Verification items for the finished model (mm, model axes). Face numbers are marked on the shaded views. A direction names the side the tool comes from. Round coordinates to 2 decimals unless told otherwise and drop trailing zeros. Order: outer loops, then holes, each group sorted by start corner. A loop starts at its lowest first (then second) coordinate and runs counter-clockwise, first axis right, second up. Notation, with made-up numbers: M 64,51.25 L 115,51.25 A17 cw 115,60.25 Z; hole C -3.5,80.25 d9. An arc over 180 degrees is marked long. One line per item, written item: value. Start each with the question number.
from build123d import *

# Parameters (mm, degrees)
SKETCH1_W           = 203.2
SKETCH1_H           = 114.3
BOSS_EXTRUDE1_DEPTH = 119.38
SHELL1_T            = -2.54
SKETCH2_R           = 18.5
SKETCH2_R_2         = 2.032
SKETCH2_R_3         = 11.176
CUT_EXTRUDE1_DEPTH  = 2.54
SKETCH3_W           = 114.3
SKETCH3_H           = 119.38
SKETCH3_R           = 18.5
SKETCH3_R_2         = 2.032
SKETCH3_R_3         = 11.176
BOSS_EXTRUDE3_DEPTH = 7.62
SKETCH4_R           = 15.875
CUT_EXTRUDE2_DEPTH  = 2.54
SKETCH5_W           = 50.7
SKETCH5_H           = 7.62
BOSS_EXTRUDE4_DEPTH = 95.25
CUT_EXTRUDE3_REACH  = 189.987
SKETCH6_R           = 3.175
FILLET1_R           = 2.54
FILLET2_R           = 2.54
SKETCH7_W           = 114.3
SKETCH7_H           = 119.38
BOSS_EXTRUDE5_DEPTH = 7.62
SKETCH8_R           = 2.54
SKETCH8_R_2         = 1.27
BOSS_EXTRUDE6_DEPTH = 5.08
SKETCH9_W           = 10.532
SKETCH9_H           = 12.532
CUT_EXTRUDE5_DEPTH  = 2.54


with BuildPart() as part:
    # Sketch1 → Boss-Extrude1 (new body)
    with BuildSketch(Plane(origin=(0, 0, 0), x_dir=(1, 0, 0), z_dir=(0, 1, 0))):
        Rectangle(SKETCH1_W, SKETCH1_H)
    extrude(amount=BOSS_EXTRUDE1_DEPTH)

    # Shell1
    shell1_openings = [part.faces().sort_by_distance(p)[0] for p in [
        (0, 119.38, 0),
    ]]
    offset(amount=SHELL1_T, openings=shell1_openings, kind=Kind.INTERSECTION)

    # Sketch2 → Cut-Extrude1 (cut)
    with BuildSketch(Plane.ZY.offset(-99.06)):
        with Locations((0, 68.58)):
            Circle(SKETCH2_R)
        with Locations((16.637, 41.275)):
            Circle(SKETCH2_R_2)
        with Locations(Location((16.637, 8.001, 0), (0, 0, 180))):
            Circle(SKETCH2_R_2)
        with Locations((-16.637, 8.001)):
            Circle(SKETCH2_R_2)
        with Locations(Location((-16.637, 41.275, 0), (0, 0, 180))):
            Circle(SKETCH2_R_2)
        with Locations((0, 24.638)):
            Circle(SKETCH2_R_3)
    extrude(amount=-CUT_EXTRUDE1_DEPTH, mode=Mode.SUBTRACT)

    # Sketch3 → Boss-Extrude3 (add)
    with BuildSketch(Plane(origin=(101.6, 0, 0), x_dir=(0, 0, -1), z_dir=(1, 0, 0))):
        with Locations((0, 59.69)):
            Rectangle(SKETCH3_W, SKETCH3_H)
        with Locations(Location((0, 68.58, 0), (0, 0, 180))):
            Circle(SKETCH3_R, mode=Mode.SUBTRACT)
        with Locations((-16.637, 8.001)):
            Circle(SKETCH3_R_2, mode=Mode.SUBTRACT)
        with Locations(Location((16.637, 8.001, 0), (0, 0, 180))):
            Circle(SKETCH3_R_2, mode=Mode.SUBTRACT)
        with Locations((16.637, 41.275)):
            Circle(SKETCH3_R_2, mode=Mode.SUBTRACT)
        with Locations(Location((-16.637, 41.275, 0), (0, 0, 180))):
            Circle(SKETCH3_R_2, mode=Mode.SUBTRACT)
        with Locations(Location((0, 24.638, 0), (0, 0, 180))):
            Circle(SKETCH3_R_3, mode=Mode.SUBTRACT)
    extrude(amount=BOSS_EXTRUDE3_DEPTH)

    # Sketch4 → Cut-Extrude2 (cut)
    with BuildSketch(Plane.XY.offset(57.15)):
        with Locations((55.88, 76.2)):
            Circle(SKETCH4_R)
    extrude(amount=-CUT_EXTRUDE2_DEPTH, mode=Mode.SUBTRACT)

    # Sketch5 → Boss-Extrude4 (add)
    with BuildSketch(Plane(origin=(0, 2.54, 0), x_dir=(1, 0, 0), z_dir=(0, 1, 0))):
        with Locations((55.88, -34.74)):
            Rectangle(SKETCH5_W, SKETCH5_H)
    extrude(amount=BOSS_EXTRUDE4_DEPTH)

    # Sketch6 → Cut-Extrude3 (cut, up to next)
    with BuildSketch(Plane.XY.offset(38.55), mode=Mode.PRIVATE) as cut_extrude3_sk1:
        with Locations((40.88, 91.2)):
            Circle(SKETCH6_R)
    cut_extrude3_tool1 = extrude(cut_extrude3_sk1.sketch, amount=-CUT_EXTRUDE3_REACH, mode=Mode.PRIVATE) & part.part
    # Sketch6 → Cut-Extrude3 (cut, up to next)
    with BuildSketch(Plane.XY.offset(38.55), mode=Mode.PRIVATE) as cut_extrude3_sk2:
        with Locations((70.88, 61.2)):
            Circle(SKETCH6_R)
    cut_extrude3_tool2 = extrude(cut_extrude3_sk2.sketch, amount=-CUT_EXTRUDE3_REACH, mode=Mode.PRIVATE) & part.part
    # Sketch6 → Cut-Extrude3 (cut, up to next)
    with BuildSketch(Plane.XY.offset(38.55), mode=Mode.PRIVATE) as cut_extrude3_sk3:
        with Locations((40.88, 61.2)):
            Circle(SKETCH6_R)
    cut_extrude3_tool3 = extrude(cut_extrude3_sk3.sketch, amount=-CUT_EXTRUDE3_REACH, mode=Mode.PRIVATE) & part.part
    # Sketch6 → Cut-Extrude3 (cut, up to next)
    with BuildSketch(Plane.XY.offset(38.55), mode=Mode.PRIVATE) as cut_extrude3_sk4:
        with Locations((70.88, 91.2)):
            Circle(SKETCH6_R)
    cut_extrude3_tool4 = extrude(cut_extrude3_sk4.sketch, amount=-CUT_EXTRUDE3_REACH, mode=Mode.PRIVATE) & part.part
    add(cut_extrude3_tool1.solids().sort_by_distance((40.88, 91.2, 38.55))[0], mode=Mode.SUBTRACT)
    add(cut_extrude3_tool2.solids().sort_by_distance((70.88, 61.2, 38.55))[0], mode=Mode.SUBTRACT)
    add(cut_extrude3_tool3.solids().sort_by_distance((40.88, 61.2, 38.55))[0], mode=Mode.SUBTRACT)
    add(cut_extrude3_tool4.solids().sort_by_distance((70.88, 91.2, 38.55))[0], mode=Mode.SUBTRACT)

    # Fillet1
    fillet1_edges = [part.edges().sort_by_distance(p)[0] for p in [
        (30.53, 97.79, 34.74),
        (81.23, 97.79, 34.74),
    ]]
    fillet(fillet1_edges, radius=FILLET1_R)

    # Fillet2
    fillet2_edges = [part.edges().sort_by_distance(p)[0] for p in [
        (30.53, 2.54, 34.74),
        (55.88, 2.54, 38.55),
        (81.23, 2.54, 34.74),
        (55.88, 2.54, 30.93),
    ]]
    fillet(fillet2_edges, radius=FILLET2_R)

    # Sketch7 → Boss-Extrude5 (add)
    with BuildSketch(Plane.ZY.offset(101.6)):
        with Locations((0, 59.69)):
            Rectangle(SKETCH7_W, SKETCH7_H)
    extrude(amount=BOSS_EXTRUDE5_DEPTH)

    # Sketch8 → Boss-Extrude6 (add)
    with BuildSketch(Plane(origin=(0, 2.54, 0), x_dir=(1, 0, 0), z_dir=(0, 1, 0))):
        with Locations(Location((57.72714395, -23.731482064, 0), (0, 0, 90))):
            Circle(SKETCH8_R)
        with Locations(Location((57.72714395, -23.731482064, 0), (0, 0, 270))):
            Circle(SKETCH8_R_2, mode=Mode.SUBTRACT)
        with Locations(Location((59.61714395, 34.233185903, 0), (0, 0, 90))):
            Circle(SKETCH8_R)
        with Locations(Location((59.61714395, 34.233185903, 0), (0, 0, 270))):
            Circle(SKETCH8_R_2, mode=Mode.SUBTRACT)
        with Locations(Location((-26.27785605, 34.233185903, 0), (0, 0, 90))):
            Circle(SKETCH8_R)
        with Locations(Location((-26.27785605, 34.233185903, 0), (0, 0, 270))):
            Circle(SKETCH8_R_2, mode=Mode.SUBTRACT)
        with Locations(Location((-28.27285605, -23.731482064, 0), (0, 0, 90))):
            Circle(SKETCH8_R)
        with Locations(Location((-28.27285605, -23.731482064, 0), (0, 0, 270))):
            Circle(SKETCH8_R_2, mode=Mode.SUBTRACT)
    extrude(amount=BOSS_EXTRUDE6_DEPTH)

    # Sketch9 → Cut-Extrude5 (cut)
    with BuildSketch(Plane(origin=(0, 0, -57.15), x_dir=(-1, 0, 0), z_dir=(0, 0, -1))):
        with Locations((-57.61714395, 14.695)):
            Rectangle(SKETCH9_W, SKETCH9_H)
        with BuildLine():
            Line((24.081592809, 9.382068871), (24.743724913, 8.719936793))
            ThreePointArc((24.743724913, 8.719936793), (25.203108007, 8.412986741), (25.744987314, 8.305200015))
            Line((25.744987314, 8.305200015), (28.362856093, 8.30520005))
            Line((28.362856093, 8.30520005), (28.402856063, 8.305200055))
            Line((28.402856063, 8.305200055), (31.020725099, 8.305200038))
            ThreePointArc((31.020725099, 8.305200038), (31.56260424, 8.412986824), (32.021987195, 8.719936816))
            Line((32.021987195, 8.719936816), (32.684119236, 9.382068816))
            ThreePointArc((32.684119236, 9.382068816), (32.991069464, 9.841452284), (33.09885605, 10.383332036))
            Line((33.09885605, 10.383332036), (33.09885605, 11.271200015))
            ThreePointArc((33.09885605, 11.271200015), (32.684119246, 12.272463208), (31.682856049, 12.687199998))
            Line((31.682856049, 12.687199998), (25.08285605, 12.687199999))
            ThreePointArc((25.08285605, 12.687199999), (24.08159283, 12.272463183), (23.66685605, 11.271199947))
            Line((23.66685605, 11.271199947), (23.66685605, 10.383332034))
            ThreePointArc((23.66685605, 10.383332034), (23.774642622, 9.841452319), (24.081592809, 9.382068871))
        make_face()
        Polygon((4.566873979, 8.528999922), (6.332856128, 8.529000057), (10.70285605, 8.529016793), (15.76285605, 8.529016793), (20.33285233, 8.529000057), (22.098848079, 8.528999922), (22.098856052, 22.594999424), (22.098856016, 23.660989296), (4.566853702, 23.660980854), (4.566856166, 22.594997652), align=None)
        with BuildLine():
            Line((-9.967143949, 25.681), (1.932856049, 25.681))
            ThreePointArc((1.932856049, 25.681), (3.07554061, 25.207684557), (3.54885605, 24.064999996))
            Line((3.54885605, 24.064999996), (3.54885605, 11.045))
            ThreePointArc((3.54885605, 11.045), (3.07554061, 9.902315442), (1.932856053, 9.429))
            Line((1.932856053, 9.429), (-9.96714395, 9.429))
            ThreePointArc((-9.96714395, 9.429), (-11.109828508, 9.902315442), (-11.58314395, 11.045000001))
            Line((-11.58314395, 11.045000001), (-11.58314395, 24.065))
            ThreePointArc((-11.58314395, 24.065), (-11.109828508, 25.207684559), (-9.967143949, 25.681))
        make_face()
        with BuildLine():
            Line((-26.967143949, 25.681), (-15.067143954, 25.681))
            ThreePointArc((-15.067143954, 25.681), (-13.924459392, 25.207684559), (-13.45114395, 24.064999998))
            Line((-13.45114395, 24.064999998), (-13.45114395, 11.044999999))
            ThreePointArc((-13.45114395, 11.044999999), (-13.924459391, 9.902315442), (-15.067143949, 9.429))
            Line((-15.067143949, 9.429), (-26.967143951, 9.429))
            ThreePointArc((-26.967143951, 9.429), (-28.109828509, 9.902315442), (-28.58314395, 11.045))
            Line((-28.58314395, 11.045), (-28.58314395, 24.065))
            ThreePointArc((-28.58314395, 24.065), (-28.109828508, 25.207684559), (-26.967143949, 25.681))
        make_face()
        with BuildLine():
            Line((-32.21714395, 27.3712), (-47.51714395, 27.3712))
            ThreePointArc((-47.51714395, 27.3712), (-48.082829375, 27.136885425), (-48.31714395, 26.5712))
            Line((-48.31714395, 26.5712), (-48.31714395, 10.168080492))
            ThreePointArc((-48.31714395, 10.168080492), (-48.229275984, 9.955948458), (-48.01714395, 9.868080492))
            Line((-48.01714395, 9.868080492), (-31.71714395, 9.868080492))
            ThreePointArc((-31.71714395, 9.868080492), (-31.527817248, 9.935367364), (-31.423418556, 10.107044492))
            Line((-31.423418556, 10.107044492), (-31.423418556, 26.6712))
            ThreePointArc((-31.423418556, 26.6712), (-31.687993687, 27.1712), (-32.21714395, 27.3712))
        make_face()
    extrude(amount=-CUT_EXTRUDE5_DEPTH, mode=Mode.SUBTRACT)


solid = part.part
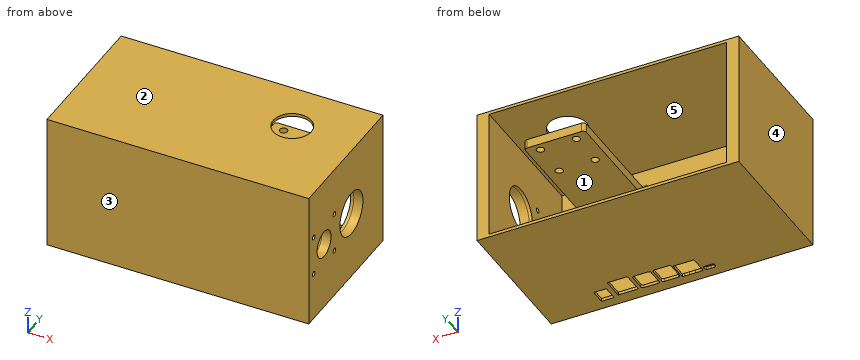
1. Section check D-D (x = 88.5). Record the cut outline in (y, z).
2. Section check B-B (z = 0). Record the cut outline in (x, y), and give its area (3 significant figures).
3. Scan lines: line 1 along Z through (x, y) = (73.5, 75); line 2 along Y through (x, z) = (107, 0); line 3 along X through (y, z) = (38.5, -32.5). Record each from-to range of solid material in increasing order.
4. Tool access check on the marked faces 4 and 5. Record the directions out of +Z, -Z, +X, -X, +Y, -Y that give a thin tool (end or side, any length) a straight path to the whole face; none if there is none.
5. Section check C-C (y = 76.2). Record the cut outline in (x, z) (3 decimals).
6. Depth check by flat-ended pin: pin 1 (5 mm diameter, centred on x = -77, z = -11.5, fed in from +Y). Enter the tip coordinate at first touch or a pass-through.
7. Draft check along Z on the marked faces 1, 2 and 3. Enter one of: released by +Z, released by -Z, zero draft, split by the parting line, or undercut.
8. Section check A-A (x = 3). Record the cut outline in (y, z).
Geometry check:
1. outline: M 0,-57.15 L 119.38,-57.15 L 119.38,-54.61 L 2.54,-54.61 L 2.54,54.61 L 119.38,54.61 L 119.38,57.15 L 0,57.15 Z
2. outline: M -109.22,0 L 109.22,0 L 109.22,13.46 L 99.06,13.46 L 99.06,2.54 L -99.06,2.54 L -99.06,119.38 L -109.22,119.38 Z; M 99.06,35.81 L 109.22,35.81 L 109.22,50.08 L 99.06,50.08 Z; M 99.06,87.08 L 109.22,87.08 L 109.22,119.38 L 99.06,119.38 Z
2. area: 2,330 mm²
3. line 1: z = -57.15 to -54.61, 30.93 to 38.55, 54.61 to 57.15
3. line 2: y = 0 to 13.46, 35.81 to 50.08, 87.08 to 119.38
3. line 3: x = -109.22 to -99.06, 99.06 to 109.22
4. face 4: +Z, -Z, -X, +Y, -Y
4. face 5: +Y
5. outline: M -109.22,-57.15 L 109.22,-57.15 L 109.22,-16.858 L 99.06,-16.858 L 99.06,-54.61 L -99.06,-54.61 L -99.06,54.61 L 40.005,54.61 L 40.005,57.15 L -109.22,57.15 Z; M 30.53,30.93 L 81.23,30.93 L 81.23,38.55 L 30.53,38.55 Z; M 71.755,54.61 L 99.06,54.61 L 99.06,16.858 L 109.22,16.858 L 109.22,57.15 L 71.755,57.15 Z
6. pin 1: stops at y = 2.54
7. face 1: undercut
7. face 2: released by +Z
7. face 3: zero draft
8. outline: M 0,-57.15 L 9.43,-57.15 L 9.43,-54.61 L 2.54,-54.61 L 2.54,54.61 L 119.38,54.61 L 119.38,57.15 L 0,57.15 Z; M 25.68,-57.15 L 119.38,-57.15 L 119.38,-54.61 L 25.68,-54.61 Z
